Source: CAD feature listing. Evaluate the final solid. Frame: model axes, mm. Face numbers are marked on the shaded views. Round coordinates to 2 decimals unless told otherwise and drop trailing zeros. Loops run counter-clockwise (first coordinate to the right, second up) from the corner with the lowest first, then second, coordinate; pieces in that order, holes last.
Item 1: Section query C-C on x = 22.5. Return loops of the section in (y, z), then the cut area to 3 significant figures.
Item 2: Pull-direction query (Z, two-part tool) for the marked faces 1, 2 and 3; classes: released by +Z, released by -Z, zero draft, split by the parting line, or undercut.
Item 3: Section query B-B on x = 0. Return loops of the section in (y, z), then the cut area to 3 significant figures.
Item 4: Ray query, L1, parallel to X at y = 12, z = 0; L2, parallel to Y at x = -23, z = 26; L3, parallel to X at y = 13, z = -34. Return the intervals inside material, ascending.
Item 5: First-contact query: P1, Ø3.5, axis at x = 22.5, z = -38.97, coming from the +Y side; P2, Ø5, axis at y = 2, z = -27, coming from the -X side; P3, Ø5.5, axis at x = 22.5, z = 38.97, coming from the +Y side; P4, Ø10, axis at x = 12.5, z = 30.5, coming from the +Y side. Flat tips, straight axial feed; report the tip coordinate or a pass-through.
Item 6: Section query A-A on y = 4.75. Give the number of separate pieces and of enclosed holes in the cut face, then the cut area to 3 significant figures.
Item 7: Section query D-D on z = -21.5. Return loops of the section in (x, y), then the cut area to 3 significant figures.
```python
from build123d import *

# Parameters (mm, degrees)
EXTRUDE_1_DEPTH     = 2.5
SKETCH_3_R          = 2.1
SKETCH_3_R_2        = 30
CUT_EXTRUDE_1_DEPTH = 2.5
EXTRUDE_START       = 13
SKETCH_4_R          = 6.15
SKETCH_4_R_2        = 2.1
EXTRUDE_2_DEPTH     = 13


with BuildPart() as part:
    # 草图2 → 凸台-拉伸1 (new body)
    with BuildSketch(Plane(origin=(0, 0, 0), x_dir=(1, 0, 0), z_dir=(0, 1, 0))):
        with BuildLine():
            ThreePointArc((32.014603848, -35.893430769), (33.749999498, -19.485572455), (47.091922833, -9.77874526))
            ThreePointArc((47.091922833, -9.77874526), (55, 8.44e-07), (47.091921183, 9.778745613))
            ThreePointArc((47.091921183, 9.778745613), (33.749999557, 19.485572352), (32.014603255, 35.893428936))
            ThreePointArc((32.014603255, 35.893428936), (27.499999447, 47.631397528), (15.077318804, 45.67217323))
            ThreePointArc((15.077318804, 45.67217323), (-6.08e-07, 38.97114317), (-15.077319619, 45.672174133))
            ThreePointArc((-15.077319619, 45.672174133), (-27.500000167, 47.631397112), (-32.014603117, 35.893428511))
            ThreePointArc((-32.014603117, 35.893428511), (-33.750000135, 19.485571351), (-47.091923006, 9.778745223))
            ThreePointArc((-47.091923006, 9.778745223), (-55, 1.241e-06), (-47.091925432, -9.778744704))
            ThreePointArc((-47.091925432, -9.778744704), (-33.7500007, -19.485570372), (-32.014603185, -35.89342872))
            ThreePointArc((-32.014603185, -35.89342872), (-27.500001103, -47.631396571), (-15.077321215, -45.672175901))
            ThreePointArc((-15.077321215, -45.672175901), (-1.245e-06, -38.97114317), (15.077319547, -45.672174053))
            ThreePointArc((15.077319547, -45.672174053), (27.499999092, -47.631397732), (32.014603848, -35.893430769))
        make_face()
    extrude(amount=EXTRUDE_1_DEPTH)

    # 草图3 → 切除-拉伸1 (cut)
    with BuildSketch(Plane(origin=(0, 2.5, 0), x_dir=(1, 0, 0), z_dir=(0, 1, 0))):
        with Locations(Location((-22.5, 38.97114317, 0), (0, 0, 270))):
            Circle(SKETCH_3_R)
        with Locations(Location((22.5, 38.97114317, 0), (0, 0, 270))):
            Circle(SKETCH_3_R)
        with Locations(Location((45, 0, 0), (0, 0, 270))):
            Circle(SKETCH_3_R)
        with Locations(Location((22.5, -38.97114317, 0), (0, 0, 270))):
            Circle(SKETCH_3_R)
        with Locations(Location((-22.5, -38.97114317, 0), (0, 0, 270))):
            Circle(SKETCH_3_R)
        with Locations(Location((-45, 0, 0), (0, 0, 270))):
            Circle(SKETCH_3_R)
        with Locations(Location((0, 0, 0), (0, 0, 270))):
            Circle(SKETCH_3_R_2)
    extrude(amount=-CUT_EXTRUDE_1_DEPTH, mode=Mode.SUBTRACT)

    # 草图4 → 凸台-拉伸2 (add)
    # profile 1 of 6: a face of its own
    with BuildSketch(Plane(origin=(0, 2.5, 0), x_dir=(1, 0, 0), z_dir=(0, 1, 0)).offset(EXTRUDE_START)):
        with Locations(Location((-22.5, 38.97114317, 0), (0, 0, 90))):
            Circle(SKETCH_4_R)
        with Locations(Location((-22.5, 38.97114317, 0), (0, 0, 270))):
            Circle(SKETCH_4_R_2, mode=Mode.SUBTRACT)
    # profile 2 of 6: a face of its own
    with BuildSketch(Plane(origin=(0, 2.5, 0), x_dir=(1, 0, 0), z_dir=(0, 1, 0)).offset(EXTRUDE_START)):
        with Locations(Location((22.5, 38.97114317, 0), (0, 0, 90))):
            Circle(SKETCH_4_R)
        with Locations(Location((22.5, 38.97114317, 0), (0, 0, 270))):
            Circle(SKETCH_4_R_2, mode=Mode.SUBTRACT)
    # profile 3 of 6: a face of its own
    with BuildSketch(Plane(origin=(0, 2.5, 0), x_dir=(1, 0, 0), z_dir=(0, 1, 0)).offset(EXTRUDE_START)):
        with Locations(Location((45, 0, 0), (0, 0, 90))):
            Circle(SKETCH_4_R)
        with Locations(Location((45, 0, 0), (0, 0, 270))):
            Circle(SKETCH_4_R_2, mode=Mode.SUBTRACT)
    # profile 4 of 6: a face of its own
    with BuildSketch(Plane(origin=(0, 2.5, 0), x_dir=(1, 0, 0), z_dir=(0, 1, 0)).offset(EXTRUDE_START)):
        with Locations(Location((22.5, -38.97114317, 0), (0, 0, 90))):
            Circle(SKETCH_4_R)
        with Locations(Location((22.5, -38.97114317, 0), (0, 0, 270))):
            Circle(SKETCH_4_R_2, mode=Mode.SUBTRACT)
    # profile 5 of 6: a face of its own
    with BuildSketch(Plane(origin=(0, 2.5, 0), x_dir=(1, 0, 0), z_dir=(0, 1, 0)).offset(EXTRUDE_START)):
        with Locations(Location((-22.5, -38.97114317, 0), (0, 0, 90))):
            Circle(SKETCH_4_R)
        with Locations(Location((-22.5, -38.97114317, 0), (0, 0, 270))):
            Circle(SKETCH_4_R_2, mode=Mode.SUBTRACT)
    # profile 6 of 6: a face of its own
    with BuildSketch(Plane(origin=(0, 2.5, 0), x_dir=(1, 0, 0), z_dir=(0, 1, 0)).offset(EXTRUDE_START)):
        with Locations(Location((-45, 0, 0), (0, 0, 90))):
            Circle(SKETCH_4_R)
        with Locations(Location((-45, 0, 0), (0, 0, 270))):
            Circle(SKETCH_4_R_2, mode=Mode.SUBTRACT)
    extrude(amount=-EXTRUDE_2_DEPTH)


solid = part.part
```
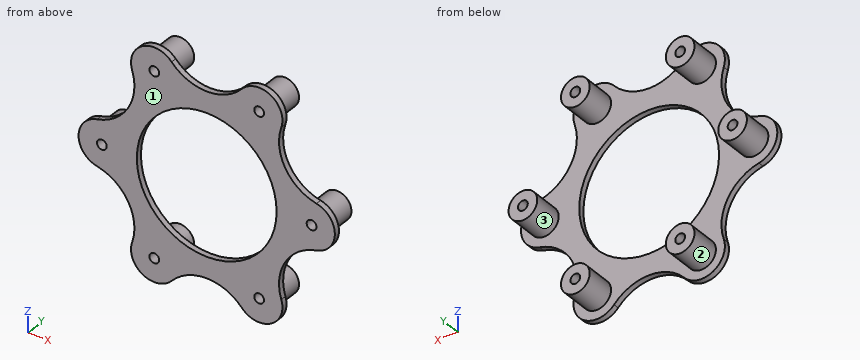
Data:
1. outline: (0, -48.97) - (2.5, -48.97) - (2.5, -45.12) - (15.5, -45.12) - (15.5, -41.07) - (0, -41.07) - close; (0, -36.87) - (15.5, -36.87) - (15.5, -32.82) - (2.5, -32.82) - (2.5, -19.84) - (0, -19.84) - close; (0, 19.84) - (2.5, 19.84) - (2.5, 32.82) - (15.5, 32.82) - (15.5, 36.87) - (0, 36.87) - close; (0, 41.07) - (15.5, 41.07) - (15.5, 45.12) - (2.5, 45.12) - (2.5, 48.97) - (0, 48.97) - close
1. area: 335 mm2
2. face 1: zero draft
2. face 2: undercut
2. face 3: split by the parting line
3. outline: (0, -38.97) - (2.5, -38.97) - (2.5, -30) - (0, -30) - close; (0, 30) - (2.5, 30) - (2.5, 38.97) - (0, 38.97) - close
3. area: 44.9 mm2
4. L1: x = -51.15 to -47.1, -42.9 to -38.85, 38.85 to 42.9, 47.1 to 51.15
4. L2: y = 0 to 2.5
4. L3: x = -26.12 to -18.88, 18.88 to 26.12
5. P1: passes through
5. P2: stops at x = -31.69
5. P3: stops at y = 15.5
5. P4: stops at y = 2.5
6. separate pieces: 6
6. enclosed holes: 6
6. area: 630 mm2
7. outline: (-32.73, 0) - (-20.92, 0) - (-20.92, 2.5) - (-32.73, 2.5) - close; (20.92, 0) - (32.73, 0) - (32.73, 2.5) - (20.92, 2.5) - close
7. area: 59.0 mm2
